Check sheet for the drawn part. Datum: minimum x, y, z corner. Units: mm. A direction names the side the tool comes from. Give positions to 0.01 mm unless a question says otherwise; leave off trailing zeros. Order: outer loops, then holes, each group sorted by start corner. A loop starts at its lowest first (then second) coordinate and runs counter-clockwise, first axis right, second up. Notation, with made-up numbers: (51.5, 6.5) - (104.5, 6.5) arc R16 cw to (104.5, 10.5) - close; hole circle Ø10 at (-8, -20.5). An arc over 180 degrees is marked (long way). Answer as a JSON object with one key per item and string values. Group by question number.
(1) Mould release check, pull along X, two halves, no side actions. Record for the marked faces 4, 5, 6 and 7: +X half, -X half, draft (parallel to the pull), parting line (faces both ways), or undercut.
(2) Section check A-A (z = 22.5). Record the boundary of the cut face in (x, y), then the cut area to 3 significant figures.
(3) Access from +Z, -Z, +X, -X, +Y, -Y to the whole of each face (thin tool, end or side, straight path). Record for the marked faces 1, 2 and 3.
(4) Section check D-D (x = 34.5). Record the boundary of the cut face in (y, z).
(5) Thickness scan on line 1 (X direction, y = 32.5, z = 24); line 2 (X direction, y = 54.5, z = 36); line 3 (X direction, y = 65, z = 6). Record the ranges inside material, lowest first.
(6) Section check B-B (y = 39). Record the boundary of the cut face in (x, z), then the cut area to 3 significant figures.
(7) Section check C-C (z = 32). Record the boundary of the cut face in (x, y), then the cut area to 3 significant figures.
(8) Depth check by flat-ended pin: pin 1 Ø2.5 at (x, y) = (57, 29.5) entering from -Z; pin 2 Ø10 at (x, y) = (39, 46) entering from -Z; pin 3 Ø4 at (y, z) = (44, 3) entering from -X. Enter the tip coordinate at first touch or a pass-through.
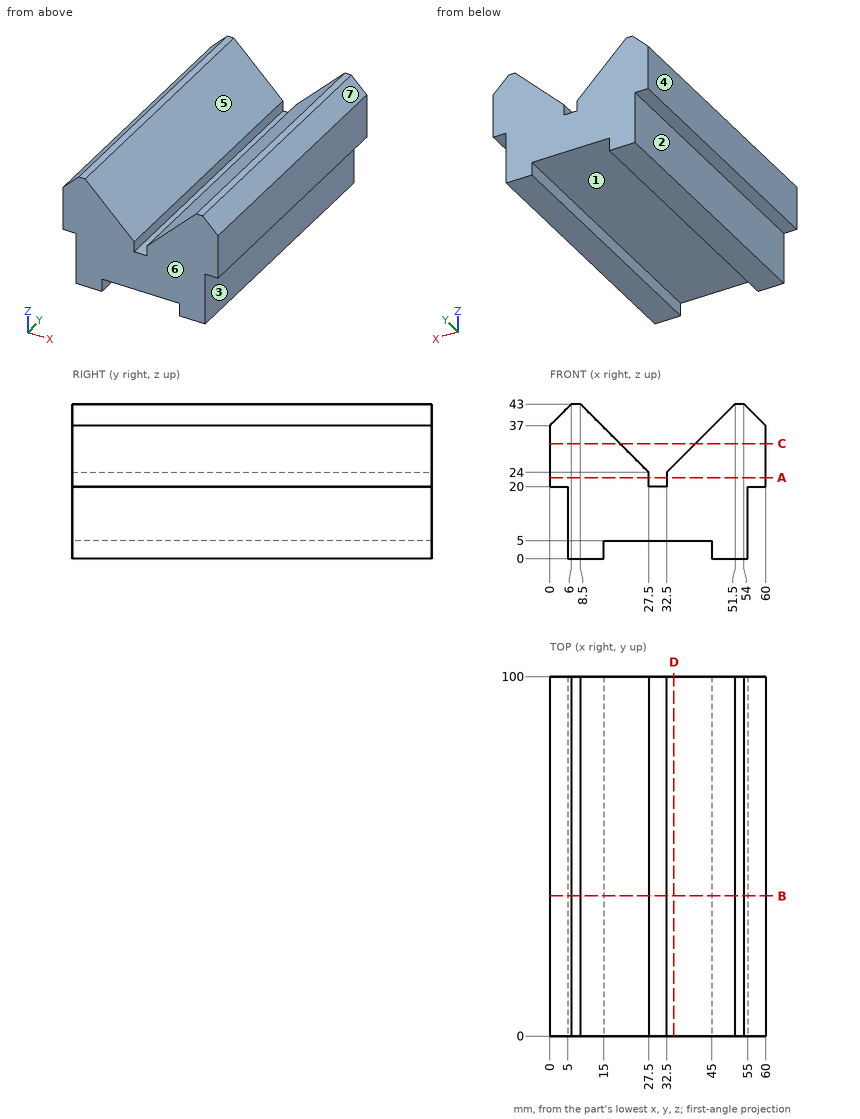
Solutions:
{
 "1": {"face 4": "-X half", "face 5": "undercut", "face 6": "draft", "face 7": "+X half"},
 "2": {"outline": "(0, 0) - (27.5, 0) - (27.5, 100) - (0, 100) - close; (32.5, 0) - (60, 0) - (60, 100) - (32.5, 100) - close", "area": "5,500 mm2"},
 "3": {"face 1": "-Z, +Y, -Y", "face 2": "-Z, -X, +Y, -Y", "face 3": "-Z, +X, +Y, -Y"},
 "4": {"outline": "(0, 5) - (100, 5) - (100, 26) - (0, 26) - close"},
 "5": {"line 1": "x = 0 to 27.5, 32.5 to 60", "line 2": "x = 0 to 15.5, 44.5 to 60", "line 3": "x = 5 to 55"},
 "6": {"outline": "(0, 20) - (5, 20) - (5, 0) - (15, 0) - (15, 5) - (45, 5) - (45, 0) - (55, 0) - (55, 20) - (60, 20) - (60, 37) - (54, 43) - (51.5, 43) - (32.5, 24) - (32.5, 20) - (27.5, 20) - (27.5, 24) - (8.5, 43) - (6, 43) - (0, 37) - close", "area": "1,720 mm2"},
 "7": {"outline": "(0, 0) - (19.5, 0) - (19.5, 100) - (0, 100) - close; (40.5, 0) - (60, 0) - (60, 100) - (40.5, 100) - close", "area": "3,900 mm2"},
 "8": {"pin 1": "stops at z = 20", "pin 2": "stops at z = 5", "pin 3": "stops at x = 5"}
}
